Could you check a few things on this drawing? It's one solid part, dimensions in mm from its lowest x, y, z. A direction names the side the tool comes from. Round coordinates to 2 decimals unless told otherwise and drop trailing zeros. Write each loop counter-clockwise with the first axis right and the second up, starting at its lowest first coordinate (ties: lowest second). Pieces come first, ordered by that corner, then holes. Notation, with made-up numbers: (11.25, 45.5) - (49.25, 45.5) arc R6 ccw to (49.25, 50.5) - close; hole circle Ø4 at (82, 45). An arc over 180 degrees is marked (long way). One line per question, with ' | ' between items. Start each with the question number.
(1) Imagine slicing it at B-B (z = 25.5). Write out the boundary of the cut face in (x, y), plus the area to 3 significant figures.
(2) Imagine slicing it at D-D (z = 16.75). Write out the boundary of the cut face in (x, y).
(3) Imagine slicing it at C-C (y = 31.75). Write out the boundary of the cut face in (x, z).
(4) For the marked faces 5, 6 and 7, which set-ups out of +Z, -Z, +X, -X, +Y, -Y let a thin tool reach every point of the face, with its end or its side?
(5) Thinking about a two-plate mould opening in Z: for the marked faces 1, 2, 3 and 4, which applies, pulls with the +Z half, pulls with the -Z half, needs draft (parallel to the pull), parting line crosses it, or undercut?
(6) Imagine slicing it at A-A (y = 5). Write out the boundary of the cut face in (x, z).
(7) Will these pins go through, and if not, where does the flat tip stop? pin 1 (7 mm diameter, centred on x = 35.5, z = 3.5, fed in from -Y); pin 2 (2 mm diameter, centred on x = 46.75, y = 31.75, fed in from +Z); pin 3 (14.5 mm diameter, centred on x = 31.75, y = 31.75, fed in from -Z).
(8) If I drill on L1, parallel to X at y = 3.25, z = 16.75; L2, parallel to Z at x = 55.5, y = 3.5; L3, parallel to Z at x = 38, y = 54.5, over which ranges is the centre line in solid material (lowest first)?
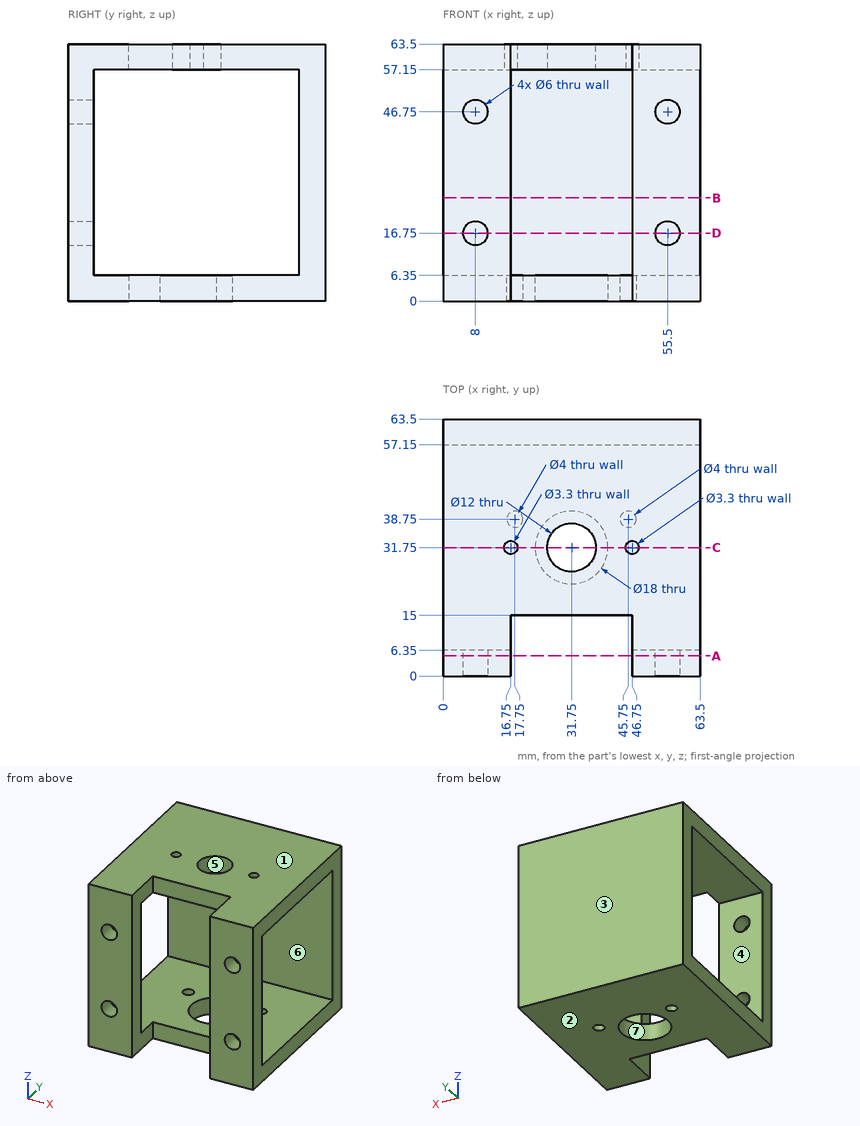
Check sheet entries:
1) outline: (0, 0) - (16.75, 0) - (16.75, 6.35) - (0, 6.35) - close; (0, 57.15) - (63.5, 57.15) - (63.5, 63.5) - (0, 63.5) - close; (46.75, 0) - (63.5, 0) - (63.5, 6.35) - (46.75, 6.35) - close | area: 616 mm^2
2) outline: (0, 0) - (5, 0) - (5, 6.35) - (0, 6.35) - close; (0, 57.15) - (63.5, 57.15) - (63.5, 63.5) - (0, 63.5) - close; (11, 0) - (16.75, 0) - (16.75, 6.35) - (11, 6.35) - close; (46.75, 0) - (52.5, 0) - (52.5, 6.35) - (46.75, 6.35) - close; (58.5, 0) - (63.5, 0) - (63.5, 6.35) - (58.5, 6.35) - close
3) outline: (0, 0) - (22.75, 0) - (22.75, 6.35) - (0, 6.35) - close; (0, 57.15) - (15.1, 57.15) - (15.1, 63.5) - (0, 63.5) - close; (18.4, 57.15) - (25.75, 57.15) - (25.75, 63.5) - (18.4, 63.5) - close; (37.75, 57.15) - (45.1, 57.15) - (45.1, 63.5) - (37.75, 63.5) - close; (40.75, 0) - (63.5, 0) - (63.5, 6.35) - (40.75, 6.35) - close; (48.4, 57.15) - (63.5, 57.15) - (63.5, 63.5) - (48.4, 63.5) - close
4) face 5: +Z, -Z | face 6: +X, -X | face 7: -Z
5) face 1: pulls with the +Z half | face 2: pulls with the -Z half | face 3: needs draft | face 4: undercut
6) outline: (0, 0) - (16.75, 0) - (16.75, 63.5) - (0, 63.5) - close; (46.75, 0) - (63.5, 0) - (63.5, 63.5) - (46.75, 63.5) - close; hole circle Ø6 at (8, 16.75); hole circle Ø6 at (8, 46.75); hole circle Ø6 at (55.5, 16.75); hole circle Ø6 at (55.5, 46.75)
7) pin 1: y = 15 | pin 2: z = 6.35 | pin 3: z = 57.15
8) L1: 0 to 5, 11 to 16.75, 46.75 to 52.5, 58.5 to 63.5 | L2: 0 to 13.75, 19.75 to 43.75, 49.75 to 63.5 | L3: 0 to 6.35, 57.15 to 63.5
